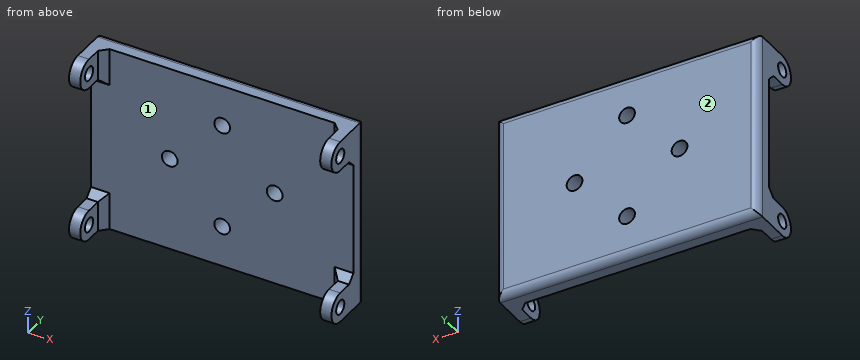
```python
from build123d import *

# Parameters (mm, degrees)
SKETCH_1_W          = 35
SKETCH_1_H          = 25
EXTRUDE_1_DEPTH     = 1.225
EXTRUDE_2_DEPTH     = 1.5
SKETCH_4_R          = 0.925
CUT_EXTRUDE_1_DEPTH = 38.682895656
CHAMFER_1_SIZE      = 1
FILLET_1_R          = 1
SKETCH_5_R          = 1.05
CUT_EXTRUDE_2_DEPTH = 23.759668275


with BuildPart() as part:
    # 草图1 → 凸台-拉伸1 (new, symmetric)
    with BuildSketch(Plane(origin=(0, 0, 0), x_dir=(1, 0, 0), z_dir=(0, 1, 0))):
        Rectangle(SKETCH_1_W, SKETCH_1_H)
    extrude(amount=EXTRUDE_1_DEPTH, both=True)

    # 草图2 → 凸台-拉伸2 (add)
    with BuildSketch(Plane.ZY.offset(17.5)):
        with BuildLine():
            Line((-12.5, -1.225), (-12.5, -4.225))
            ThreePointArc((-12.5, -4.225), (-10.5, -6.225), (-8.5, -4.225))
            Line((-8.5, -4.225), (-8.5, -1.225))
            Line((-8.5, -1.225), (-12.5, -1.225))
        make_face()
        with BuildLine():
            Line((8.5, -1.225), (12.5, -1.225))
            Line((12.5, -1.225), (12.5, -4.225))
            ThreePointArc((12.5, -4.225), (10.5, -6.225), (8.5, -4.225))
            Line((8.5, -4.225), (8.5, -1.225))
        make_face()
    extrude_2 = extrude(amount=-EXTRUDE_2_DEPTH)

    # 草图4 → 切除-拉伸1 (cut, through all)
    with BuildSketch(Plane.ZY.offset(17.5)):
        with Locations((-10.5, -4.225)):
            Circle(SKETCH_4_R)
        with Locations(Location((10.5, -4.225, 0), (0, 0, 180))):
            Circle(SKETCH_4_R)
    cut_extrude_1 = extrude(amount=-CUT_EXTRUDE_1_DEPTH, mode=Mode.SUBTRACT)

    # 镜向1: 凸台-拉伸2, 切除-拉伸1 across plane
    add(extrude_2.mirror(Plane(origin=(0, 0, 0), x_dir=(0, 0, 1), z_dir=(1, 0, 0))))
    add(cut_extrude_1.mirror(Plane(origin=(0, 0, 0), x_dir=(0, 0, 1), z_dir=(1, 0, 0))), mode=Mode.SUBTRACT)

    # 倒角1
    chamfer_1_edges = [part.edges().sort_by_distance(p)[0] for p in [
        (-16, -1.225, -10.5),
        (-16.75, -1.225, -8.5),
        (-16, -1.225, 10.5),
        (-16.75, -1.225, 8.5),
        (16.75, -1.225, -8.5),
        (16, -1.225, -10.5),
        (16.75, -1.225, 8.5),
        (16, -1.225, 10.5),
    ]]
    chamfer(chamfer_1_edges, length=CHAMFER_1_SIZE)

    # 圆角1
    fillet_1_edges = [part.edges().sort_by_distance(p)[0] for p in [
        (-17.5, 1.225, 0),
        (0, 1.225, 12.5),
        (17.5, 1.225, 0),
        (0, 1.225, -12.5),
    ]]
    fillet(fillet_1_edges, radius=FILLET_1_R)

    # 草图5 → 切除-拉伸2 (cut, through all)
    with BuildSketch(Plane(origin=(0, 1.225, 0), x_dir=(1, 0, 0), z_dir=(0, 1, 0))):
        with Locations(Location((0, 7, 0), (0, 0, 270))):
            Circle(SKETCH_5_R)
        with Locations(Location((7, 0, 0), (0, 0, 270))):
            Circle(SKETCH_5_R)
        with Locations(Location((-7, 0, 0), (0, 0, 270))):
            Circle(SKETCH_5_R)
        with Locations(Location((0, -7, 0), (0, 0, 270))):
            Circle(SKETCH_5_R)
    extrude(amount=-CUT_EXTRUDE_2_DEPTH, mode=Mode.SUBTRACT)


solid = part.part
```
Verification items for the finished model (mm, model axes). Face numbers are marked on the shaded views. Round coordinates to 2 decimals unless told otherwise and drop trailing zeros. Write each loop counter-clockwise with the first axis right and the second up, starting at its lowest first coordinate (ties: lowest second). Pieces come first, ordered by that corner, then holes. Notation, with made-up numbers: (12, -18) -> (55, -18) arc R29 cw to (55, 4) -> close; hole circle Ø8 at (56.5, 88.5). An arc over 180 degrees is marked (long way). Write each question's results on one line, items separated by ' | '.
Q1. Go/stop test with flat-tipped pins: pin 1 Ø2.5 at (x, z) = (0, 7) entering from +Y (3 decimals); pin 2 Ø1 at (x, z) = (1.5, -1.5) entering from -Y (3 decimals). Record where each tip stops, or that it passes through.
Derived:
pin 1: stops at y = 1.225 | pin 2: stops at y = -1.225
Q2. Sectioned sample at B-B, the plane x = -7. Record the boundary of the cut face in (y, z) (3 decimals), and give its area (3 significant figures).
Derived:
outline: (-1.225, -12.5) -> (0.225, -12.5) arc R1 ccw to (1.225, -11.5) -> (1.225, -1.05) -> (-1.225, -1.05) -> close; (-1.225, 1.05) -> (1.225, 1.05) -> (1.225, 11.5) arc R1 ccw to (0.225, 12.5) -> (-1.225, 12.5) -> close | area: 55.7 mm²
Q3. Sectioned sample at D-D, the plane y = -0.25. Record the boundary of the cut face in (x, z).
Derived:
outline: (-17.5, -12.5) -> (17.5, -12.5) -> (17.5, 12.5) -> (-17.5, 12.5) -> close; hole circle Ø2.1 at (-7, 0); hole circle Ø2.1 at (0, -7); hole circle Ø2.1 at (0, 7); hole circle Ø2.1 at (7, 0)
Q4. Sectioned sample at C-C, the plane z = -7. Record the boundary of the cut face in (x, y) (3 decimals), and give its area (3 significant figures).
Derived:
outline: (-17.5, -1.225) -> (-1.05, -1.225) -> (-1.05, 1.225) -> (-16.5, 1.225) arc R1 ccw to (-17.5, 0.225) -> close; (1.05, -1.225) -> (17.5, -1.225) -> (17.5, 0.225) arc R1 ccw to (16.5, 1.225) -> (1.05, 1.225) -> close | area: 80.2 mm²
Q5. Draft check along Z on the marked faces 1 and 2. Enter one of: released by +Z, released by -Z, zero draft, split by the parting line, or undercut.
Derived:
face 1: undercut | face 2: zero draft
Q6. Thickness scan on probe 1 along Y at (x, z) = (16.4, -10.5) (3 decimals); probe 2 along X at (y, z) = (0.3, -7); probe 3 along X at (y, z) = (-3.5, 9). Record the ranges inside material, lowest first.
Derived:
probe 1: y = -6.225 to -5.15, -3.3 to 1.225 | probe 2: x = -17.5 to -1.05, 1.05 to 17.5 | probe 3: x = -17.5 to -16, 16 to 17.5
Q7. Sectioned sample at A-A, the plane z = 10.5. Record the boundary of the cut face in (x, y) (3 decimals).
Derived:
outline: (-17.5, -6.225) -> (-16, -6.225) -> (-16, -5.15) -> (-17.5, -5.15) -> close; (-17.5, -3.3) -> (-16, -3.3) -> (-16, -2.225) -> (-15, -1.225) -> (15, -1.225) -> (16, -2.225) -> (16, -3.3) -> (17.5, -3.3) -> (17.5, 0.225) arc R1 ccw to (16.5, 1.225) -> (-16.5, 1.225) arc R1 ccw to (-17.5, 0.225) -> close; (16, -6.225) -> (17.5, -6.225) -> (17.5, -5.15) -> (16, -5.15) -> close
